```python
from build123d import *

# Parameters (mm, degrees)
F0_W     = 10
F0_H     = 40
F1_DEPTH = 30
F2_R     = 4.99999
F3_R     = 5
F4_DEPTH = 5
F5_W     = 30
F5_H     = 30
F6_DEPTH = 30
F7_R     = 14.99999


# Not quite as in the source:
# - a fillet or chamfer is up to 0.001 mm smaller than in the source, because OpenCascade refuses the exact size


with BuildPart() as f1:
    # F0 (on Right) → F1 (new body)
    with BuildSketch(Plane.YZ):
        with Locations((5, 20)):
            Rectangle(F0_W, F0_H)
    extrude(amount=-F1_DEPTH)

    # F2 (radius 5 in the source; OpenCascade refuses exactly that, so slightly less here)
    f2_edges = [f1.edges().sort_by_distance(p)[0] for p in [
        (0, 10, 20),
        (0, 0, 20),
        (-30, 10, 20),
        (-30, 0, 20),
    ]]
    fillet(f2_edges, radius=F2_R)

    # F3 (on face) → F4 (join)
    with BuildSketch(Plane.XY.offset(40)):
        with Locations((-15, 5)):
            Circle(F3_R)
    extrude(amount=F4_DEPTH)

    # F5 (on face) → F6 (join)
    with BuildSketch(Plane.XY.offset(45)):
        with Locations((-15, 7.1624371922)):
            Rectangle(F5_W, F5_H)
    extrude(amount=F6_DEPTH)

    # F7 (radius 15 in the source; OpenCascade refuses exactly that, so slightly less here)
    f7_edges = [f1.edges().sort_by_distance(p)[0] for p in [
        (-15, -7.837563, 75),
        (0, 7.162437, 75),
        (-15, 22.162437, 75),
        (-30, 7.162437, 75),
        (-30, 22.162437, 60),
        (0, 22.162437, 60),
        (0, -7.837563, 60),
        (-30, -7.837563, 60),
    ]]
    fillet(f7_edges, radius=F7_R)


solid = f1.part
```
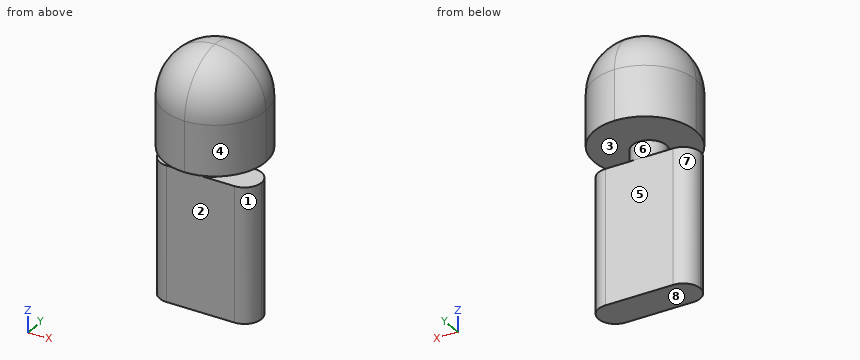
Design review of the part built by this model. Coordinates are the model's own, in mm. Face numbers are marked on the shaded views. A direction names the side the tool comes from. Give positions to 0.01 mm unless a question says otherwise; leave off trailing zeros. Return JSON: item names as keys, results as strings. Group by question number.
Item 1: Mouldability with a two-part tool opening along Z and no side actions: class the marked faces 6, 7 and 8 as released by +Z, released by -Z, zero draft, split by the parting line, or undercut.
Item 2: Insertion check: pin 1 Ø3 at (x, z) = (-20, 19.5) entering from -Y; pin 2 Ø1 at (x, y) = (-6, 2) entering from +Z; pin 3 Ø8 at (x, y) = (-6, 3) entering from +Z; pin 4 Ø15 at (x, y) = (-12, 8.5) entering from -Z. Each pin has a flat end and moves straight along its axis. Give the tip position at first contact, or say it passes through.
Item 3: For probe 1 along Y at (x, z) = (-7, 21); probe 2 along Z at (x, y) = (-22, 3.5); probe 3 along Z at (x, y) = (-3, 1), list the stretches that pass through material, from the lowest coordinate up.
Item 4: Tool access review of the marked faces 1, 2, 3, 4 and 5: name each direction out of +Z, -Z, +X, -X, +Y, -Y from which nothing blocks a thin tool from reaching the whole face with its end or side.
Output:
{
 "1": {"face 6": "undercut", "face 7": "zero draft", "face 8": "released by -Z"},
 "2": {"pin 1": "stops at y = 0", "pin 2": "stops at z = 71.29", "pin 3": "stops at z = 73.78", "pin 4": "stops at z = 0"},
 "3": {"probe 1": "y = 0 to 10", "probe 2": "z = 0 to 40, 45 to 72.75", "probe 3": "z = 0 to 40, 45 to 66.56"},
 "4": {"face 1": "-Z, +X, -Y", "face 2": "-Z, +X, -X, -Y", "face 3": "+X, +Y", "face 4": "+Z, +X, -Y", "face 5": "-Z, +X, -X, +Y"}
}
